from build123d import *

# Parameters (mm, degrees)
SKETCH_1_W      = 27
SKETCH_1_H      = 9
SKETCH_1_H_2    = 1.4
BOTTOM_DEPTH    = 1.4
SKETCH_1_3_W    = 27
SKETCH_1_3_H    = 1.4
EXTRUDE_2_DEPTH = 8


with BuildPart() as part:
    # Sketch 1 → Bottom (new body)
    with BuildSketch(Plane(origin=(0, 0, 0), x_dir=(1, 0, 0), z_dir=(0, 1, 0))):
        with Locations((13.5, 5.9)):
            Rectangle(SKETCH_1_W, SKETCH_1_H)
        with Locations((13.5, 11.1)):
            Rectangle(SKETCH_1_W, SKETCH_1_H_2)
        with Locations((13.5, 0.7)):
            Rectangle(SKETCH_1_W, SKETCH_1_H_2)
    extrude(amount=BOTTOM_DEPTH)

    # Sketch 1_3 → Extrude 2 (add)
    with BuildSketch(Plane(origin=(0, 0, 0), x_dir=(1, 0, 0), z_dir=(0, 1, 0))):
        with Locations((13.5, 11.1)):
            Rectangle(SKETCH_1_3_W, SKETCH_1_3_H)
        with Locations((13.5, 0.7)):
            Rectangle(SKETCH_1_3_W, SKETCH_1_3_H)
    extrude(amount=EXTRUDE_2_DEPTH)


solid = part.part
Input: part model. Units: mm. Frame: model coordinates. A direction names the side the tool comes from. Coordinates: 2 decimals unless noted, no trailing zeros. Loops run counter-clockwise (first coordinate to the right, second up) from the corner with the lowest first, then second, coordinate; pieces in that order, holes last.
Q1. Material intervals for line 1 (Z direction, x = 16.5, y = 2.5); line 2 (Y direction, x = 7.5, z = -4), sorted ascending.
Q2. Contact query for a flat-ended pin moving along its axis: pin 1 (1 mm diameter, centred on y = 2, z = -9, fed in from +X). Output: stop coordinate, or through.
Q3. Set-up query: faces 4 (the face through (13, 1.4, -6)), 5 (the face through (13, 8, -11)). Return all of +Z, -Z, +X, -X, +Y, -Y with unobstructed straight access to the full face (end or side cutting, diameter ignored); none if empty.
Q4. Cut plane B-B (x = 7.25). Output: boundary loops of the cut face in (y, z).
Q5. Cut plane A-A (y = 5). Output: boundary loops of the cut face in (x, z).
Q6. Draft query along Z for faces 1 (the face through (13, 4, -11.8)), 2 (the face through (13, 5, -1.4)), 3 (the face through (13, 8, -1)). Return one class per face: +Z half, -Z half, draft (parallel to the pull), parting line (faces both ways), or undercut.
Q7. Cut plane C-C (z = -6). Output: boundary loops of the cut face in (x, y).
Working result:
1. line 1: z = -11.8 to -10.4, -1.4 to 0
1. line 2: y = 0 to 1.4
2. pin 1: passes through
3. face 4: +X, -X, +Y
3. face 5: +Z, -Z, +X, -X, +Y
4. outline: (0, -11.8) - (8, -11.8) - (8, -10.4) - (1.4, -10.4) - (1.4, -1.4) - (8, -1.4) - (8, 0) - (0, 0) - close
5. outline: (0, -11.8) - (27, -11.8) - (27, -10.4) - (0, -10.4) - close; (0, -1.4) - (27, -1.4) - (27, 0) - (0, 0) - close
6. face 1: -Z half
6. face 2: undercut
6. face 3: draft
7. outline: (0, 0) - (27, 0) - (27, 1.4) - (0, 1.4) - close
